Read the model definition and answer for the solid it produces. Units are mm, in the model's axes. Face numbers are marked on the shaded views. Give positions to 0.01 mm unless a question says otherwise; leave off trailing zeros. Write each loop counter-clockwise with the first axis right and the second up, starting at its lowest first coordinate (ties: lowest second). Pieces come first, ordered by that corner, then holes. Notation, with made-up numbers: M 42.25,-26.75 L 69.25,-26.75 A25 ccw 69.25,-11.75 Z; hole C -0.5,-8.5 d3. An arc over 180 degrees is marked long. Put each result on its own line as item: value.
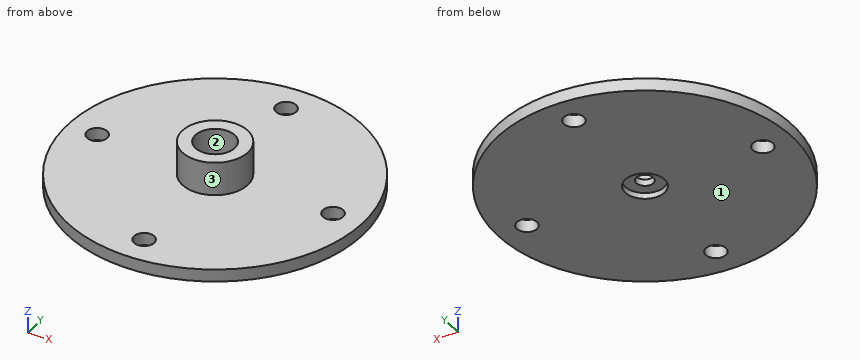
from build123d import *

# Parameters (mm, degrees)
F0_R     = 22.5
F0_R_2   = 1.55
F0_R_3   = 5
F1_DEPTH = 1.9
F0_R_4   = 3
F2_DEPTH = 7
F3_START = 0.9
F0_R_5   = 1.3
F3_DEPTH = 1


with BuildPart() as f1:
    # F0 (on Top) → F1 (new body)
    with BuildSketch(Plane.XY):
        Circle(F0_R)
        with Locations((0, -18)):
            Circle(F0_R_2, mode=Mode.SUBTRACT)
        with Locations((-18, 0)):
            Circle(F0_R_2, mode=Mode.SUBTRACT)
        Circle(F0_R_3, mode=Mode.SUBTRACT)
        with Locations((18, 0)):
            Circle(F0_R_2, mode=Mode.SUBTRACT)
        with Locations((0, 18)):
            Circle(F0_R_2, mode=Mode.SUBTRACT)
    extrude(amount=F1_DEPTH)

    # F0 (on Top) → F2 (join)
    with BuildSketch(Plane.XY):
        Circle(F0_R_3)
        Circle(F0_R_4, mode=Mode.SUBTRACT)
    extrude(amount=F2_DEPTH)

    # F0 (on Top) → F3 (join)
    with BuildSketch(Plane.XY.offset(F3_START)):
        Circle(F0_R_4)
        Circle(F0_R_5, mode=Mode.SUBTRACT)
    extrude(amount=F3_DEPTH)


solid = f1.part
(1) Section A-A on x = 18 is taken. Determine the outline of the cut face in (y, z).
Result:
outline: M -13.5,0 L -1.55,0 L -1.55,1.9 L -13.5,1.9 Z; M 1.55,0 L 13.5,0 L 13.5,1.9 L 1.55,1.9 Z
(2) Section B-B on y = 0 is taken. Determine the outline of the cut face in (x, z), and give its area (3 significant figures).
Result:
outline: M -22.5,0 L -19.55,0 L -19.55,1.9 L -22.5,1.9 Z; M -16.45,0 L -3,0 L -3,0.9 L -1.3,0.9 L -1.3,1.9 L -3,1.9 L -3,7 L -5,7 L -5,1.9 L -16.45,1.9 Z; M 1.3,0.9 L 3,0.9 L 3,0 L 16.45,0 L 16.45,1.9 L 5,1.9 L 5,7 L 3,7 L 3,1.9 L 1.3,1.9 Z; M 19.55,0 L 22.5,0 L 22.5,1.9 L 19.55,1.9 Z
area: 86.1 mm²
(3) For a pull along Y with two mould halves and no side action, classify the marked faces 1, 2 and 3 as +Y half, -Y half, draft (parallel to the pull), parting line (faces both ways), or undercut.
Result:
face 1: draft
face 2: undercut
face 3: parting line
(4) Given pin 1 Ø2 at (y, z) = (3, 3.5) entering from +X; pin 2 Ø3 at (x, y) = (0, -1) entering from -Z; pin 3 Ø3.5 at (x, y) = (18, 0) entering from +Z, each flat-ended and moving along its own axis, determine where each tip first touches the part or whether it passes through.
Result:
pin 1: stops at x = 4.58
pin 2: stops at z = 0.9
pin 3: stops at z = 1.9
(5) Straight lines are drawn through the part: line 1 along Y through (x, z) = (0, 1.6); line 2 along Y through (x, z) = (0, 0.3); line 3 along Y through (x, z) = (0, 3.95). For each, find the intervals that lie inside material, in ascending order. Write a range as from..to.
Result:
line 1: y = -22.5..-19.55, -16.45..-1.3, 1.3..16.45, 19.55..22.5
line 2: y = -22.5..-19.55, -16.45..-3, 3..16.45, 19.55..22.5
line 3: y = -5..-3, 3..5
